```python
from build123d import *

# Parameters (mm, degrees)
F0_R         = 30
F1_DEPTH     = 20
F2_R         = 21.9
F3_DEPTH     = 5
F4_R         = 20
F5_DEPTH     = 42
F6_R         = 21.7
F6_R_2       = 20
F7_DEPTH     = 3
F9_D         = 10
F9_DEPTH     = 80
F9_TIP       = 3.0043030951
F11_D        = 10
F11_DEPTH    = 50
F11_TIP      = 3.0043030951
F12_S5_R     = 20
F12_T6_DEPTH = 32


# Not quite as in the source:
# - a fillet or chamfer that OpenCascade refuses, or shapes differently, is made with other operations: its cross-section is extruded or revolved along the edge and cut away or added


with BuildPart() as f1:
    # F0 (on Top) → F1 (new body)
    with BuildSketch(Plane.XY):
        Circle(F0_R)
        with BuildLine():
            ThreePointArc((14.4568322948, -4), (-15, 0), (14.4568322948, 4))
            Line((14.4568322948, 4), (18, 4))
            Line((18, 4), (18, 0))
            Line((18, 0), (18, -4))
            Line((18, -4), (14.4568322948, -4))
        make_face(mode=Mode.SUBTRACT)
    extrude(amount=F1_DEPTH)

    # F2 (on face) → F3 (join)
    with BuildSketch(Plane.XY.offset(20)):
        Circle(F2_R)
        with BuildLine():
            ThreePointArc((14.4568322948, -4), (-15, 0), (14.4568322948, 4))
            Line((14.4568322948, 4), (18, 4))
            Line((18, 4), (18, -4))
            Line((18, -4), (14.4568322948, -4))
        make_face(mode=Mode.SUBTRACT)
    extrude(amount=F3_DEPTH)

    # F4 (on face) → F5 (join)
    with BuildSketch(Plane.XY.offset(25)):
        Circle(F4_R)
        with BuildLine():
            ThreePointArc((14.4568322948, -4), (-15, 0), (14.4568322948, 4))
            Line((14.4568322948, 4), (18, 4))
            Line((18, 4), (18, -4))
            Line((18, -4), (14.4568322948, -4))
        make_face(mode=Mode.SUBTRACT)
    extrude(amount=F5_DEPTH)

    # F6 (on face) → F7 (join)
    with BuildSketch(Plane.XY.offset(67)):
        Circle(F6_R)
        Circle(F6_R_2, mode=Mode.SUBTRACT)
        Circle(F6_R_2)
        with BuildLine():
            ThreePointArc((14.4568322948, -4), (-15, 0), (14.4568322948, 4))
            Line((14.4568322948, 4), (18, 4))
            Line((18, 4), (18, -4))
            Line((18, -4), (14.4568322948, -4))
        make_face(mode=Mode.SUBTRACT)
    extrude(amount=F7_DEPTH)

    # F9 (one way)
    with BuildSketch(Plane(origin=(0, 0, 0), x_dir=(0, 1, 0), z_dir=(-1, 0, 0))):
        with Locations((0, -10)):
            Circle(F9_D / 2)
    extrude(amount=-F9_DEPTH, mode=Mode.SUBTRACT)
    with Locations(Plane(origin=(0, 0, 0), x_dir=(0, 1, 0), z_dir=(-1, 0, 0))):
        with Locations((0, -10)):
            with Locations((0, 0, -(F9_DEPTH + F9_TIP / 2))):  # 118° drill point
                Cone(0, F9_D / 2, F9_TIP, mode=Mode.SUBTRACT)

    # F11 (one way)
    with BuildSketch(Plane.XZ):
        with Locations((0, 10)):
            Circle(F11_D / 2)
    extrude(amount=-F11_DEPTH, mode=Mode.SUBTRACT)
    with Locations(Plane.XZ):
        with Locations((0, 10)):
            with Locations((0, 0, -(F11_DEPTH + F11_TIP / 2))):  # 118° drill point
                Cone(0, F11_D / 2, F11_TIP, mode=Mode.SUBTRACT)

    # F12: chamfer of 2 on 1 edges, made by hand


with BuildPart() as f12_tool2:
    # F12_s3 → F12_t4 (revolve)
    with BuildSketch(Plane.XZ):
        Polygon((21.9, 23), (19.9, 25), (21.9, 25), align=None)
    revolve(axis=Axis((0, 0, 25), (0, 0, 1)))

    # F12_s5 → F12_t6 (cut, symmetric)
    with BuildSketch(Plane.XY.offset(24)):
        Circle(F12_S5_R)
    extrude(amount=F12_T6_DEPTH, both=True, mode=Mode.SUBTRACT)


with BuildPart() as f1_1:
    add(f1.part)

    # F12_t1: cut F12_tool2
    add(f12_tool2.part, mode=Mode.SUBTRACT)


solid = f1_1.part
```
Can you work these out from the model? Positions are in its coordinate system, mm. A direction names the side the tool comes from. Round coordinates to 2 decimals unless told otherwise and drop trailing zeros. Order: outer loops, then holes, each group sorted by start corner. A loop starts at its lowest first (then second) coordinate and runs counter-clockwise, first axis right, second up. Notation, with made-up numbers: (36.25, -28) -> (44.25, -28) arc R12 ccw to (44.25, -5) -> close; hole circle Ø7 at (13, 75). An arc over 180 degrees is marked (long way). Return JSON: item names as keys, results as strings. Group by question number.
1. We'd pull the mould along X, two halves only. Please class faces 4 (the face through (16, 4, 41)), 5 (the face through (-14.988, -0.603, 34.51)), 6 (the face through (10, -18, 67)), 7 (the face through (-15.99, 14.67, 68.48)): released by +X, released by -X, zero draft, split by the parting line, or undercut.
2. If we section it at D-D, the plane z = 10: Write out the boundary of the cut face in (x, y), then the cut area to 3 significant figures.
3. If we section it at C-C, the plane z = 27: Write out the boundary of the cut face in (x, y).
4. Which directions (+Z, -Z, +X, -X, +Y, -Y) give clear straight access to the entire face, cutting with the end or side of a thin tool? Please do faces 1 (the face through (4.77, 21.96, 11.5)), 2 (the face through (18, 0, 41)), 3 (the face through (-17.4, -13.3, 21.5)).
5. If we section it at B-B, the plane x = 0: Write out the boundary of the cut face in (y, z), then the cut area to 3 significant figures.
6. If we section it at A-A, the plane y = 0: Write out the boundary of the cut face in (x, z), then the cut area to 3 significant figures.
7. Will these pins go through, and if not, where does the flat tip stop? pin 1 (12 mm diameter, centred on x = 16, z = 35.5, fed in from -Y); pin 2 (6 mm diameter, centred on x = 0, z = 10, fed in from +Y); pin 3 (1.5 mm diameter, centred on x = 19.5, y = -22.5, fed in from +Z); pin 4 (5 mm diameter, centred on x = 24, z = 51.5, fed in from +Y).
8. I need wall thicknesses on line 1 (Y direction, x = 0, z = 50); line 2 (Z direction, x = 0, y = 21.5); line 3 (Z direction, x = 19, y = 0). Which ranges of each line are inside material? Lowest first, please. Write a range as [from, to].
Output values:
{
 "1": {"face 4": "undercut", "face 5": "undercut", "face 6": "zero draft", "face 7": "split by the parting line"},
 "2": {"outline": "(-5, 14.14) -> (-5, 29.58) arc R30 ccw (long way) to (29.58, -5) -> (14.14, -5) arc R15 cw (long way) to start; (5, 14.14) arc R15 cw to (14.14, 5) -> (29.58, 5) arc R30 ccw to (5, 29.58) -> close", "area": "1,820 mm²"},
 "3": {"outline": "circle Ø40 at (0, 0); hole (14.46, -4) -> (18, -4) -> (18, 4) -> (14.46, 4) arc R15 ccw (long way) to start"},
 "4": {"face 1": "+Y", "face 2": "+Z, -Z", "face 3": "+Z"},
 "5": {"outline": "(-30, 0) -> (-15, 0) -> (-15, 70) -> (-21.7, 70) -> (-21.7, 67) -> (-20, 67) -> (-20, 24.9) -> (-21.9, 23) -> (-21.9, 20) -> (-30, 20) -> close; (15, 0) -> (30, 0) -> (30, 5) -> (15, 5) -> close; (15, 15) -> (30, 15) -> (30, 20) -> (21.9, 20) -> (21.9, 23) -> (20, 24.9) -> (20, 67) -> (21.7, 67) -> (21.7, 70) -> (15, 70) -> close", "area": "975 mm²"},
 "6": {"outline": "(-30, 0) -> (-15, 0) -> (-15, 70) -> (-21.7, 70) -> (-21.7, 67) -> (-20, 67) -> (-20, 24.9) -> (-21.9, 23) -> (-21.9, 20) -> (-30, 20) -> close; (18, 0) -> (30, 0) -> (30, 5) -> (18, 5) -> close; (18, 15) -> (30, 15) -> (30, 20) -> (21.9, 20) -> (21.9, 23) -> (20, 24.9) -> (20, 67) -> (21.7, 67) -> (21.7, 70) -> (18, 70) -> close", "area": "795 mm²"},
 "7": {"pin 1": "y = -17.32", "pin 2": "y = -14.7", "pin 3": "z = 20", "pin 4": "through"},
 "8": {"line 1": "[-20, -15], [15, 20]", "line 2": "[0, 5], [15, 23.4], [67, 70]", "line 3": "[0, 5], [15, 70]"}
}
